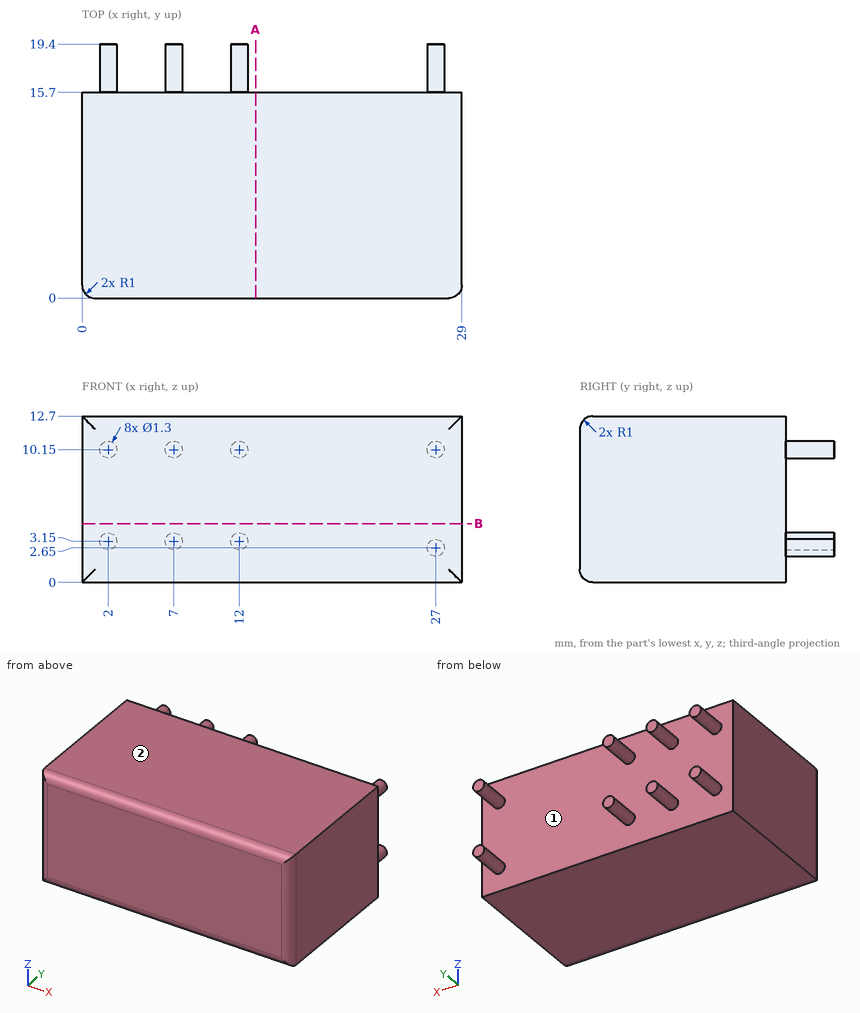
Geometry check sheet. Reference: drawing and pictorial views, mm from the part's lowest x, y, z. A direction names the side the tool comes from. Round coordinates to 2 decimals unless told otherwise and drop trailing zeros. Loops run counter-clockwise (first coordinate to the right, second up) from the corner with the lowest first, then second, coordinate; pieces in that order, holes last. Notation, with made-up numbers: M -29,-17 L 23,-17 A13 ccw 23,-7 Z; hole C 88.25,59 d4. An arc over 180 degrees is marked long. One line per item, written item: value.
(1) Sectioned sample at B-B, the plane z = 4.5. Record the cut outline in (x, y), then the cut area to 3 significant figures.
Computed values:
outline: M 0,1 A1 ccw 1,0 L 28,0 A1 ccw 29,1 L 29,15.7 L 0,15.7 Z
area: 455 mm^2
(2) Sectioned sample at A-A, the plane x = 13.25. Record the cut outline in (y, z), then the cut area to 3 significant figures.
Computed values:
outline: M 0,1 A1 ccw 1,0 L 15.7,0 L 15.7,12.7 L 1,12.7 A1 ccw 0,11.7 Z
area: 199 mm^2
(3) Thickness scan on line 1 (Y direction, x = 8.75, z = 9). Record the ranges inside material, lowest first.
Computed values:
line 1: y = 0 to 15.7
(4) Depth check by flat-ended pin: pin 1 Ø3 at (x, z) = (21.5, 1.5) entering from +Y. Enter the tip coordinate at first touch or a pass-through.
Computed values:
pin 1: stops at y = 15.7
(5) Access from +Z, -Z, +X, -X, +Y, -Y to the whole of each face (thin tool, end or side, straight path). Record for the marked faces 1 and 2.
Computed values:
face 1: +Y
face 2: +Z, +X, -X, +Y, -Y
